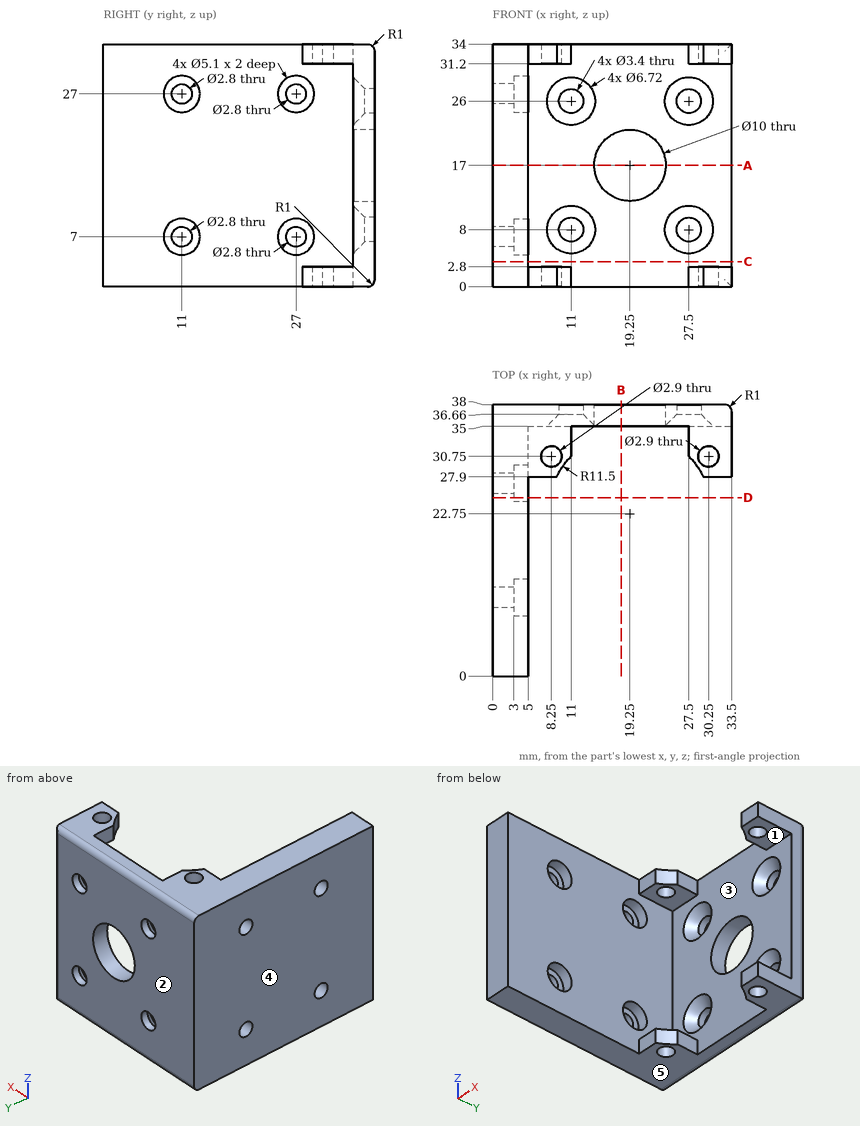
Study the drawing (mm; zero at the part's minimum x, y, z) and answer. A direction names the side the tool comes from. Coordinates: 2 decimals unless noted, no trailing zeros. Loops run counter-clockwise (first coordinate to the right, second up) from the corner with the lowest first, then second, coordinate; pieces in that order, holes last. Notation, with made-up numbers: (14.25, 31) -> (44.25, 31) arc R22 cw to (44.25, 56) -> close; hole circle Ø11 at (30.25, 57.5). An arc over 180 degrees is marked (long way). Answer as CSV lines item,"result".
1) For the marked faces 1 and 2, determine the directions among +Z, -Z, +X, -X, +Y, -Y from which every point of the face is accessible in a straight line to the end or side of a thin tool.
A:
face 1,"+X, -Y"
face 2,"+Z, -Z, +X, -X, +Y"
2) For a pull along Z with two mould halves and no side action, classify the marked faces 3, 4 and 5 as released by +Z, released by -Z, zero draft, split by the parting line, or undercut.
A:
face 3,"undercut"
face 4,"zero draft"
face 5,"released by -Z"
3) The part is cut by section D-D (y = 25). Give the vertices of the cut face in (x, z).
A:
outline,"(0, 0) -> (5, 0) -> (5, 5.42) -> (3, 5.42) -> (3, 8.58) -> (5, 8.58) -> (5, 25.42) -> (3, 25.42) -> (3, 28.58) -> (5, 28.58) -> (5, 34) -> (0, 34) -> close"
4) The part is cut by section C-C (z = 3.5). Give the vertices of the cut face in (x, y), and give its area (3 significant figures).
A:
outline,"(0, 0) -> (5, 0) -> (5, 35) -> (33.5, 35) -> (33.5, 37) arc R1 ccw to (32.5, 38) -> (0, 38) -> close"
area,"275 mm²"
5) Straight lines are drawn through the part: probe 1 along Z at (x, y) = (2.4, 11); probe 2 along Y at (x, z) = (24, 32.5); probe 3 along X at (y, z) = (7, 6.5). For each, find the intervals that lie inside material, in ascending order.
A:
probe 1,"z = 0 to 5.6, 8.4 to 25.6, 28.4 to 34"
probe 2,"y = 35 to 38"
probe 3,"x = 0 to 5"
6) The part is cut by section A-A (z = 17). Give the vertices of the cut face in (x, y), and give its area (3 significant figures).
A:
outline,"(0, 0) -> (5, 0) -> (5, 35) -> (14.25, 35) -> (14.25, 38) -> (0, 38) -> close; (24.25, 35) -> (33.5, 35) -> (33.5, 37) arc R1 ccw to (32.5, 38) -> (24.25, 38) -> close"
area,"245 mm²"
7) The part is cut by section B-B (x = 18). Give the vertices of the cut face in (y, z).
A:
outline,"(35, 0) -> (37, 0) arc R1 ccw to (38, 1) -> (38, 12.16) -> (35, 12.16) -> close; (35, 21.84) -> (38, 21.84) -> (38, 33) arc R1 ccw to (37, 34) -> (35, 34) -> close"
8) Flat-ended cylindrical pins translate along their axes: pin 1 (2 mm diameter, centred on x = 32.5, z = 1, fed in from -Y); pin 2 (2 mm diameter, centred on y = 27, z = 27, fed in from -X); pin 3 (10 mm diameter, centred on y = 17.5, z = 14, fed in from +X). Find the tip coordinate at first contact, or state that the pin passes through.
A:
pin 1,"stops at y = 27.9"
pin 2,"passes through"
pin 3,"stops at x = 5"
